Could you check a few things on this model? Use its own coordinates, in mm. A direction names the side the tool comes from. Coordinates: 2 decimals unless noted, no trailing zeros. Write each loop counter-clockwise with the first axis right and the second up, starting at its lowest first coordinate (ties: lowest second). Pieces come first, ordered by that corner, then holes. Notation, with made-up numbers: M -13.5,71 L 20.5,71 A33 cw 20.5,109 Z; hole C 25.25,34 d3. An arc over 180 degrees is marked long. Write item = value, one per line.
```python
from build123d import *

# Parameters (mm, degrees)
BOSS_EXTRUDE1_DEPTH = 4
SKETCH1_3_R         = 1.6
BOSS_EXTRUDE2_DEPTH = 2


with BuildPart() as part:
    # Sketch1 → Boss-Extrude1 (new body)
    with BuildSketch(Plane.XY):
        with BuildLine():
            Line((66.665147012, 36.773979945), (37.187967483, 36.773979945))
            ThreePointArc((37.187967483, 36.773979945), (36.122555312, 36.447160452), (35.42366679, 35.579134584))
            ThreePointArc((35.42366679, 35.579134584), (32.126890988, 33.777131531), (29.734357819, 36.673979945))
            ThreePointArc((29.734357819, 36.673979945), (29.177860704, 38.017482829), (27.834357819, 38.573979945))
            Line((27.834357819, 38.573979945), (-20.554852988, 38.573979945))
            ThreePointArc((-20.554852988, 38.573979945), (-21.898355872, 38.017482829), (-22.454852988, 36.673979945))
            ThreePointArc((-22.454852988, 36.673979945), (-23.318887983, 34.58801494), (-25.404852988, 33.723979945))
            ThreePointArc((-25.404852988, 33.723979945), (-26.748355872, 33.167482829), (-27.304852988, 31.823979945))
            Line((-27.304852988, 31.823979945), (-27.304852988, -11.034660039))
            ThreePointArc((-27.304852988, -11.034660039), (-26.748355872, -12.378162923), (-25.404852988, -12.934660039))
            ThreePointArc((-25.404852988, -12.934660039), (-22.454852988, -15.884660039), (-25.404852988, -18.834660039))
            ThreePointArc((-25.404852988, -18.834660039), (-26.748355872, -19.391157155), (-27.304852988, -20.734660039))
            Line((-27.304852988, -20.734660039), (-27.304852988, -47.916020055))
            ThreePointArc((-27.304852988, -47.916020055), (-26.748355872, -49.259522939), (-25.404852988, -49.816020055))
            ThreePointArc((-25.404852988, -49.816020055), (-23.318887983, -50.680055051), (-22.454852988, -52.766020055))
            ThreePointArc((-22.454852988, -52.766020055), (-21.898355872, -54.109522939), (-20.554852988, -54.666020055))
            Line((-20.554852988, -54.666020055), (18.205147012, -54.666020055))
            ThreePointArc((18.205147012, -54.666020055), (19.548649897, -54.109522939), (20.105147012, -52.766020055))
            ThreePointArc((20.105147012, -52.766020055), (23.055147012, -49.816020055), (26.005147012, -52.766020055))
            ThreePointArc((26.005147012, -52.766020055), (26.561644128, -54.109522939), (27.905147012, -54.666020055))
            Line((27.905147012, -54.666020055), (66.665147012, -54.666020055))
            ThreePointArc((66.665147012, -54.666020055), (68.008649897, -54.109522939), (68.565147012, -52.766020055))
            ThreePointArc((68.565147012, -52.766020055), (69.429182008, -50.680055051), (71.515147012, -49.816020055))
            ThreePointArc((71.515147012, -49.816020055), (72.858649897, -49.259522939), (73.415147012, -47.916020055))
            Line((73.415147012, -47.916020055), (73.415147012, -13.796020055))
            ThreePointArc((73.415147012, -13.796020055), (72.858649897, -12.452517171), (71.515147012, -11.896020055))
            ThreePointArc((71.515147012, -11.896020055), (68.565147012, -8.946020055), (71.515147012, -5.996020055))
            ThreePointArc((71.515147012, -5.996020055), (72.858649897, -5.439522939), (73.415147012, -4.096020055))
            Line((73.415147012, -4.096020055), (73.415147012, 30.023979945))
            ThreePointArc((73.415147012, 30.023979945), (72.858649897, 31.367482829), (71.515147012, 31.923979945))
            ThreePointArc((71.515147012, 31.923979945), (69.429182008, 32.78801494), (68.565147012, 34.873979945))
            ThreePointArc((68.565147012, 34.873979945), (68.008649897, 36.217482829), (66.665147012, 36.773979945))
        make_face()
        with BuildLine():
            Line((66.665147012, 35.423979945), (43.986531464, 35.423979945))
            Line((43.986531464, 35.423979945), (43.986531464, 4.777360506))
            Line((43.986531464, 4.777360506), (72.065147012, 4.777360506))
            Line((72.065147012, 4.777360506), (72.065147012, 30.023979945))
            ThreePointArc((72.065147012, 30.023979945), (71.904055742, 30.412888675), (71.515147012, 30.573979945))
            ThreePointArc((71.515147012, 30.573979945), (68.474587853, 31.833420786), (67.215147012, 34.873979945))
            ThreePointArc((67.215147012, 34.873979945), (67.054055742, 35.262888675), (66.665147012, 35.423979945))
        make_face(mode=Mode.SUBTRACT)
        with BuildLine():
            Line((72.065147012, -13.796020055), (72.065147012, -47.916020055))
            ThreePointArc((72.065147012, -47.916020055), (71.904055742, -48.304928785), (71.515147012, -48.466020055))
            ThreePointArc((71.515147012, -48.466020055), (68.474587853, -49.725460896), (67.215147012, -52.766020055))
            ThreePointArc((67.215147012, -52.766020055), (67.054055742, -53.154928785), (66.665147012, -53.316020055))
            Line((66.665147012, -53.316020055), (43.986531464, -53.316020055))
            Line((43.986531464, -53.316020055), (43.986531464, 3.427360506))
            Line((43.986531464, 3.427360506), (72.065147012, 3.427360506))
            Line((72.065147012, 3.427360506), (72.065147012, -4.096020055))
            ThreePointArc((72.065147012, -4.096020055), (71.904055742, -4.484928785), (71.515147012, -4.646020055))
            ThreePointArc((71.515147012, -4.646020055), (67.215147012, -8.946020055), (71.515147012, -13.246020055))
            ThreePointArc((71.515147012, -13.246020055), (71.904055742, -13.407111325), (72.065147012, -13.796020055))
        make_face(mode=Mode.SUBTRACT)
        with BuildLine():
            Line((27.905147012, -53.316020055), (42.636531464, -53.316020055))
            Line((42.636531464, -53.316020055), (42.636531464, 3.427360506))
            Line((42.636531464, 3.427360506), (17.844811896, 3.427360506))
            Line((17.844811896, 3.427360506), (17.844811896, -53.316020055))
            Line((17.844811896, -53.316020055), (18.205147012, -53.316020055))
            ThreePointArc((18.205147012, -53.316020055), (18.594055742, -53.154928785), (18.755147012, -52.766020055))
            ThreePointArc((18.755147012, -52.766020055), (23.055147012, -48.466020055), (27.355147012, -52.766020055))
            ThreePointArc((27.355147012, -52.766020055), (27.516238283, -53.154928785), (27.905147012, -53.316020055))
        make_face(mode=Mode.SUBTRACT)
        with BuildLine():
            Line((-20.554852988, -53.316020055), (16.494811896, -53.316020055))
            Line((16.494811896, -53.316020055), (16.494811896, 3.427360506))
            Line((16.494811896, 3.427360506), (-25.954852988, 3.427360506))
            Line((-25.954852988, 3.427360506), (-25.954852988, -11.034660039))
            ThreePointArc((-25.954852988, -11.034660039), (-25.793761717, -11.423568769), (-25.404852988, -11.584660039))
            ThreePointArc((-25.404852988, -11.584660039), (-21.104852988, -15.884660039), (-25.404852988, -20.184660039))
            ThreePointArc((-25.404852988, -20.184660039), (-25.793761717, -20.34575131), (-25.954852988, -20.734660039))
            Line((-25.954852988, -20.734660039), (-25.954852988, -47.916020055))
            ThreePointArc((-25.954852988, -47.916020055), (-25.793761717, -48.304928785), (-25.404852988, -48.466020055))
            ThreePointArc((-25.404852988, -48.466020055), (-22.364293829, -49.725460896), (-21.104852988, -52.766020055))
            ThreePointArc((-21.104852988, -52.766020055), (-20.943761717, -53.154928785), (-20.554852988, -53.316020055))
        make_face(mode=Mode.SUBTRACT)
        with BuildLine():
            Line((-25.954852988, 31.823979945), (-25.954852988, 4.777360506))
            Line((-25.954852988, 4.777360506), (16.494811896, 4.777360506))
            Line((16.494811896, 4.777360506), (16.494811896, 37.223979945))
            Line((16.494811896, 37.223979945), (-20.554852988, 37.223979945))
            ThreePointArc((-20.554852988, 37.223979945), (-20.943761717, 37.062888675), (-21.104852988, 36.673979945))
            ThreePointArc((-21.104852988, 36.673979945), (-22.364293829, 33.633420786), (-25.404852988, 32.373979945))
            ThreePointArc((-25.404852988, 32.373979945), (-25.793761717, 32.212888675), (-25.954852988, 31.823979945))
        make_face(mode=Mode.SUBTRACT)
        with BuildLine():
            Line((42.636531464, 35.423979945), (42.636531464, 4.777360506))
            Line((42.636531464, 4.777360506), (17.844811896, 4.777360506))
            Line((17.844811896, 4.777360506), (17.844811896, 37.223979945))
            Line((17.844811896, 37.223979945), (27.834357819, 37.223979945))
            ThreePointArc((27.834357819, 37.223979945), (28.223266549, 37.062888675), (28.384357819, 36.673979945))
            ThreePointArc((28.384357819, 36.673979945), (31.871779048, 32.451455139), (36.677248861, 35.078103656))
            ThreePointArc((36.677248861, 35.078103656), (36.879558697, 35.329374302), (37.187967483, 35.423979945))
            Line((37.187967483, 35.423979945), (42.636531464, 35.423979945))
        make_face(mode=Mode.SUBTRACT)
    extrude(amount=-BOSS_EXTRUDE1_DEPTH)

    # Sketch1<3> → Boss-Extrude2 (add)
    with BuildSketch(Plane.XY):
        with BuildLine():
            Line((28.129942232, 45.773979945), (-22.043203519, 45.773979945))
            ThreePointArc((-22.043203519, 45.773979945), (-22.808570384, 45.62173901), (-23.457417081, 45.188193507))
            Line((-23.457417081, 45.188193507), (-28.61906655, 40.026544038))
            ThreePointArc((-28.61906655, 40.026544038), (-29.052612053, 39.377697341), (-29.204852988, 38.612330476))
            Line((-29.204852988, 38.612330476), (-29.204852988, -52.766020055))
            ThreePointArc((-29.204852988, -52.766020055), (-28.091858756, -55.453025824), (-25.404852988, -56.566020055))
            Line((-25.404852988, -56.566020055), (71.515147012, -56.566020055))
            ThreePointArc((71.515147012, -56.566020055), (74.202152781, -55.453025824), (75.315147012, -52.766020055))
            Line((75.315147012, -52.766020055), (75.315147012, 34.873979945))
            ThreePointArc((75.315147012, 34.873979945), (74.202152781, 37.560985714), (71.515147012, 38.673979945))
            Line((71.515147012, 38.673979945), (36.886796481, 38.673979945))
            ThreePointArc((36.886796481, 38.673979945), (36.121429616, 38.82622088), (35.472582919, 39.259766383))
            Line((35.472582919, 39.259766383), (29.544155794, 45.188193507))
            ThreePointArc((29.544155794, 45.188193507), (28.895309096, 45.62173901), (28.129942232, 45.773979945))
        make_face()
        with Locations((-25.404852988, 36.673979945)):
            Circle(SKETCH1_3_R, mode=Mode.SUBTRACT)
        with Locations((-25.404852988, -15.884660039)):
            Circle(SKETCH1_3_R, mode=Mode.SUBTRACT)
        with Locations((-25.404852988, -52.766020055)):
            Circle(SKETCH1_3_R, mode=Mode.SUBTRACT)
        with Locations((23.055147012, -52.766020055)):
            Circle(SKETCH1_3_R, mode=Mode.SUBTRACT)
        with Locations((32.684357819, 36.673979945)):
            Circle(SKETCH1_3_R, mode=Mode.SUBTRACT)
        with Locations((71.515147012, 34.873979945)):
            Circle(SKETCH1_3_R, mode=Mode.SUBTRACT)
        with Locations((71.515147012, -8.946020055)):
            Circle(SKETCH1_3_R, mode=Mode.SUBTRACT)
        with Locations((71.515147012, -52.766020055)):
            Circle(SKETCH1_3_R, mode=Mode.SUBTRACT)
    extrude(amount=BOSS_EXTRUDE2_DEPTH)


solid = part.part
```
Item 1: If I drill on line 1 along X through (y, z) = (-24.5, -0.2); line 2 along Y through (x, z) = (4.5, -1.95); line 3 along Y through (x, z) = (48.5, -2.15), over which ranges is the centre line in solid material (lowest first)?
Numbers:
line_1 = -27.3 to -25.95, 16.49 to 17.84, 42.64 to 43.99, 72.07 to 73.42
line_2 = -54.67 to -53.32, 3.43 to 4.78, 37.22 to 38.57
line_3 = -54.67 to -53.32, 3.43 to 4.78, 35.42 to 36.77
Item 2: If we mould it in two halves opening along X, with no side actions, what happens to faces 1 (the face through (30, 4.777, -2)), 2 (the face through (22.85, -51.18, 0.99)), 3 (the face through (23, -49, -4)), 4 (the face through (73.415, -31, -2))? For each: pulls with the +X half, pulls with the -X half, needs draft (parallel to the pull), parting line crosses it, or undercut.
Numbers:
face_1 = undercut
face_2 = undercut
face_3 = needs draft
face_4 = pulls with the +X half
Item 3: Imagine slicing it at C-C (y = -36). Write out the boundary of the cut face in (x, z).
Numbers:
outline = M -29.2,0 L -27.3,0 L -27.3,-4 L -25.95,-4 L -25.95,0 L 16.49,0 L 16.49,-4 L 17.84,-4 L 17.84,0 L 42.64,0 L 42.64,-4 L 43.99,-4 L 43.99,0 L 72.07,0 L 72.07,-4 L 73.42,-4 L 73.42,0 L 75.32,0 L 75.32,2 L -29.2,2 Z
Item 4: For faces 5 (the face through (73.415, 13, -2)), 6 (the face through (-21.106, -15.79, -1.972)), 7 (the face through (-22.456, -15.82, -1.972)), 8 (the face through (22.99, -49.817, -1.972)), which set-ups out of +Z, -Z, +X, -X, +Y, -Y let a thin tool reach every point of the face, with its end or its side?
Numbers:
face_5 = -Z, +X, +Y, -Y
face_6 = -Z
face_7 = -Z, -X
face_8 = -Z, -Y
Item 5: Imagine slicing it at A-A (x = 13). Write out the boundary of the cut face in (y, z), and give its area (3 significant figures).
Numbers:
outline = M -56.57,0 L -54.67,0 L -54.67,-4 L -53.32,-4 L -53.32,0 L 3.43,0 L 3.43,-4 L 4.78,-4 L 4.78,0 L 37.22,0 L 37.22,-4 L 38.57,-4 L 38.57,0 L 45.77,0 L 45.77,2 L -56.57,2 Z
area = 221 mm²
Item 6: I'm going to push flat-ended pins straight in: P1, Ø3.5, axis at x = 71.52, y = -8.95, coming from the -Z side; P2, Ø1.2, axis at y = -18.5, z = -2.5, coming from the -X side; P3, Ø1.6, axis at x = 53.5, z = 1, coming from the +Y side. Where does each tip first touch, or does it pass through?
Numbers:
P1 = 0
P2 = -26.37
P3 = 38.67
Item 7: Imagine slicing it at B-B (z = 1). State how many separate pieces and enclosed holes the cut face has, and give its area (3 significant figures).
Numbers:
separate_pieces = 1
enclosed_holes = 8
area = 10,300 mm²
